```python
from build123d import *

# Parameters (mm, degrees)
SKETCH001_W     = 0.5
SKETCH001_H     = 0.5
PAD_DEPTH       = 27.5
SKETCH002_W     = 1
SKETCH002_H     = 6.098212
POCKET_DEPTH    = 5
SKETCH003_W     = 0.5
SKETCH003_H     = 0.5
POCKET001_DEPTH = 2.7
SKETCH004_W     = 0.5
SKETCH004_H     = 0.5
POCKET002_DEPTH = 1.6


with BuildPart() as part:
    # Sketch → Revolution (revolve)
    with BuildSketch(Plane.XY):
        with BuildLine():
            ThreePointArc((4, 7), (2.828427, 9.828427), (0, 11))
            Line((0, 0), (0, 11))
            Line((4.6, 0), (0, 0))
            Line((4.6, 1), (4.6, 0))
            Line((4, 1), (4.6, 1))
            Line((4, 7), (4, 1))
        make_face()
    revolve(axis=Axis((0, 0, 0), (0, 1, 0)))

    # Sketch001 (on Face2 of Revolution) → Pad (new body)
    with BuildSketch(Plane.XZ):
        with Locations((0.635, 0)):
            Rectangle(SKETCH001_W, SKETCH001_H)
        with Locations((1.905, 0)):
            Rectangle(SKETCH001_W, SKETCH001_H)
        with Locations((-0.635, 0)):
            Rectangle(SKETCH001_W, SKETCH001_H)
        with Locations((-1.905, 0)):
            Rectangle(SKETCH001_W, SKETCH001_H)
    extrude(amount=PAD_DEPTH)

    # Sketch002 (on Face5 of Pad) → Pocket (cut)
    with BuildSketch(Plane.XZ):
        with Locations((4.5, 0)):
            Rectangle(SKETCH002_W, SKETCH002_H)
    extrude(amount=-POCKET_DEPTH, mode=Mode.SUBTRACT)

    # Sketch003 (on Face23 of Pocket) → Pocket001 (cut)
    with BuildSketch(Plane.XZ.offset(27.5)):
        with Locations((-1.905, 0)):
            Rectangle(SKETCH003_W, SKETCH003_H)
    extrude(amount=-POCKET001_DEPTH, mode=Mode.SUBTRACT)

    # Sketch004 (on Face24 of Pocket001) → Pocket002 (cut)
    with BuildSketch(Plane.XZ.offset(27.5)):
        with Locations((-0.635, 0)):
            Rectangle(SKETCH004_W, SKETCH004_H)
        with Locations((1.905, 0)):
            Rectangle(SKETCH004_W, SKETCH004_H)
    extrude(amount=-POCKET002_DEPTH, mode=Mode.SUBTRACT)


solid = part.part
```
Can you work these out from the model? Positions are in its coordinate system, mm. Give positions to 0.01 mm unless a question says otherwise; leave off trailing zeros. Write each loop counter-clockwise with the first axis right and the second up, starting at its lowest first coordinate (ties: lowest second). Pieces come first, ordered by that corner, then holes. Notation, with made-up numbers: (11, 51.5) - (21, 51.5) arc R10 ccw to (21, 67.5) - close; hole circle Ø5 at (2, 81). An arc over 180 degrees is marked (long way). Write item = value, one per line. Start each with the question number.
1. Imagine slicing it at A-A (y = -18). Please give me the cut outline in (x, z) (3 decimals).
2. Imagine slicing it at B-B (y = 2.5). Please give me the cut outline in (x, z).
3. Thinking about a two-plate mould opening in Z: for faces 1 (the face through (4, 0.5, 0)), 2 (the face through (-4.597, 0.493, -0.169)), which applies, released by +Z, released by -Z, zero draft, split by the parting line, or undercut?
4. Please list where these lines run through material, in increasing order: line 1 (Y direction, x = -2.5, z = -3.5); line 2 (Z direction, x = -0.5, y = -4); line 3 (X direction, y = 7, z = -3).
5. For pin 1 (5 mm diameter, centred on x = -0.5, y = -15.5, fed in from +Z); pin 2 (0.6 mm diameter, centred on y = -20, z = 0, fed in from +X) (3 decimals); pin 3 (2 mm diameter, centred on x = 1.5, y = 3, fed in from +Z), each with a flat end and sliding along its axis, tell me the tip position at first contact or that it passes through.
Worked answers:
q1.outline = (-2.155, -0.25) - (-1.655, -0.25) - (-1.655, 0.25) - (-2.155, 0.25) - close; (-0.885, -0.25) - (-0.385, -0.25) - (-0.385, 0.25) - (-0.885, 0.25) - close; (0.385, -0.25) - (0.885, -0.25) - (0.885, 0.25) - (0.385, 0.25) - close; (1.655, -0.25) - (2.155, -0.25) - (2.155, 0.25) - (1.655, 0.25) - close
q2.outline = circle Ø8 at (0, 0)
q3.face_1 = zero draft
q3.face_2 = split by the parting line
q4.line_1 = 0 to 1
q4.line_2 = -0.25 to 0.25
q4.line_3 = -2.65 to 2.65
q5.pin_1 = 0.25
q5.pin_2 = 2.155
q5.pin_3 = 3.97
